```python
from build123d import *

# Parameters (mm, degrees)
SKETCH_1_R          = 30
EXTRUDE_1_DEPTH     = 10
CUT_EXTRUDE_1_REACH = 45.589
SKETCH_2_R          = 1.8
SKETCH_3_R          = 3.25
CUT_EXTRUDE_2_DEPTH = 5
CUT_EXTRUDE_3_REACH = 45.589
SKETCH_4_R          = 1.8
SKETCH_5_R          = 3.15
CUT_EXTRUDE_4_DEPTH = 3
CUT_EXTRUDE_5_REACH = 45.589
SKETCH_6_R          = 11
CUT_EXTRUDE_START   = -5
CUT_EXTRUDE_6_DEPTH = 5


# Read off the part's stored shape, not the designer's step: 切除-拉伸6
with BuildPart() as part:
    # 草图1 → 凸台-拉伸1 (new body)
    with BuildSketch(Plane.XY):
        Circle(SKETCH_1_R)
    extrude(amount=EXTRUDE_1_DEPTH)

    # 草图2 → 切除-拉伸1 (cut, up to next)
    with BuildSketch(Plane.XY.offset(10), mode=Mode.PRIVATE) as cut_extrude_1_sk1:
        with Locations((0, 14)):
            Circle(SKETCH_2_R)
    cut_extrude_1_tool1 = extrude(cut_extrude_1_sk1.sketch, amount=-CUT_EXTRUDE_1_REACH, mode=Mode.PRIVATE) & part.part
    # 草图2 → 切除-拉伸1 (cut, up to next)
    with BuildSketch(Plane.XY.offset(10), mode=Mode.PRIVATE) as cut_extrude_1_sk2:
        with Locations((12.124355653, -7)):
            Circle(SKETCH_2_R)
    cut_extrude_1_tool2 = extrude(cut_extrude_1_sk2.sketch, amount=-CUT_EXTRUDE_1_REACH, mode=Mode.PRIVATE) & part.part
    # 草图2 → 切除-拉伸1 (cut, up to next)
    with BuildSketch(Plane.XY.offset(10), mode=Mode.PRIVATE) as cut_extrude_1_sk3:
        with Locations((-12.124355653, -7)):
            Circle(SKETCH_2_R)
    cut_extrude_1_tool3 = extrude(cut_extrude_1_sk3.sketch, amount=-CUT_EXTRUDE_1_REACH, mode=Mode.PRIVATE) & part.part
    add(cut_extrude_1_tool1.solids().sort_by_distance((0, 14, 10))[0], mode=Mode.SUBTRACT)
    add(cut_extrude_1_tool2.solids().sort_by_distance((12.124356, -7, 10))[0], mode=Mode.SUBTRACT)
    add(cut_extrude_1_tool3.solids().sort_by_distance((-12.124356, -7, 10))[0], mode=Mode.SUBTRACT)

    # 草图3 → 切除-拉伸2 (cut)
    with BuildSketch(Plane(origin=(0, 0, 0), x_dir=(-1, 0, 0), z_dir=(0, 0, -1))):
        with Locations((0, 14)):
            Circle(SKETCH_3_R)
        with Locations((12.125855653, -6.999133975)):
            Circle(SKETCH_3_R)
        with Locations((-12.122855653, -7.000866025)):
            Circle(SKETCH_3_R)
    extrude(amount=-CUT_EXTRUDE_2_DEPTH, mode=Mode.SUBTRACT)

    # 草图4 → 切除-拉伸3 (cut, up to next)
    with BuildSketch(Plane.XY.offset(10), mode=Mode.PRIVATE) as cut_extrude_3_sk1:
        with Locations((-15, -20)):
            Circle(SKETCH_4_R)
    cut_extrude_3_tool1 = extrude(cut_extrude_3_sk1.sketch, amount=-CUT_EXTRUDE_3_REACH, mode=Mode.PRIVATE) & part.part
    # 草图4 → 切除-拉伸3 (cut, up to next)
    with BuildSketch(Plane.XY.offset(10), mode=Mode.PRIVATE) as cut_extrude_3_sk2:
        with Locations((15, -20)):
            Circle(SKETCH_4_R)
    cut_extrude_3_tool2 = extrude(cut_extrude_3_sk2.sketch, amount=-CUT_EXTRUDE_3_REACH, mode=Mode.PRIVATE) & part.part
    # 草图4 → 切除-拉伸3 (cut, up to next)
    with BuildSketch(Plane.XY.offset(10), mode=Mode.PRIVATE) as cut_extrude_3_sk3:
        with Locations((15, 20)):
            Circle(SKETCH_4_R)
    cut_extrude_3_tool3 = extrude(cut_extrude_3_sk3.sketch, amount=-CUT_EXTRUDE_3_REACH, mode=Mode.PRIVATE) & part.part
    # 草图4 → 切除-拉伸3 (cut, up to next)
    with BuildSketch(Plane.XY.offset(10), mode=Mode.PRIVATE) as cut_extrude_3_sk4:
        with Locations((-15, 20)):
            Circle(SKETCH_4_R)
    cut_extrude_3_tool4 = extrude(cut_extrude_3_sk4.sketch, amount=-CUT_EXTRUDE_3_REACH, mode=Mode.PRIVATE) & part.part
    add(cut_extrude_3_tool1.solids().sort_by_distance((-15, -20, 10))[0], mode=Mode.SUBTRACT)
    add(cut_extrude_3_tool2.solids().sort_by_distance((15, -20, 10))[0], mode=Mode.SUBTRACT)
    add(cut_extrude_3_tool3.solids().sort_by_distance((15, 20, 10))[0], mode=Mode.SUBTRACT)
    add(cut_extrude_3_tool4.solids().sort_by_distance((-15, 20, 10))[0], mode=Mode.SUBTRACT)

    # 草图5 → 切除-拉伸4 (cut)
    with BuildSketch(Plane.XY.offset(10)):
        with Locations((-15, 20)):
            Circle(SKETCH_5_R)
        with Locations((15, 20)):
            Circle(SKETCH_5_R)
        with Locations((15, -20)):
            Circle(SKETCH_5_R)
        with Locations((-15, -20)):
            Circle(SKETCH_5_R)
    extrude(amount=-CUT_EXTRUDE_4_DEPTH, mode=Mode.SUBTRACT)

    # 草图6 → 切除-拉伸5 (cut, up to next)
    with BuildSketch(Plane.XY.offset(10), mode=Mode.PRIVATE) as cut_extrude_5_sk1:
        Circle(SKETCH_6_R)
    cut_extrude_5_tool1 = extrude(cut_extrude_5_sk1.sketch, amount=-CUT_EXTRUDE_5_REACH, mode=Mode.PRIVATE) & part.part
    add(cut_extrude_5_tool1.solids().sort_by_distance((0, 0, 10))[0], mode=Mode.SUBTRACT)

    # 切除-拉伸6 outline → 切除-拉伸6 (cut)
    with BuildSketch(Plane(origin=(0, 0, 0), x_dir=(-1, 0, 0), z_dir=(0, 0, -1)).offset(CUT_EXTRUDE_START)):
        with BuildLine():
            Line((-10.725995825, -2.439879827), (-13.749355653, -4.185417438))
            ThreePointArc((-13.749355653, -4.185417438), (-15.374355624, -7.000433013), (-13.748605595, -9.815015475))
            ThreePointArc((-13.748605595, -9.815015475), (-14.784005692, -5.135181039), (-10.031538938, -4.513117164))
            ThreePointArc((-10.031538938, -4.513117164), (-10.430407021, -3.493795841), (-10.725995825, -2.439879827))
        make_face()
        with BuildLine():
            Line((-3.25, 14), (-3.25, 10.508924778))
            ThreePointArc((-3.25, 10.508924778), (-2.189145313, 10.779964879), (-1.10660044, 10.944196429))
            ThreePointArc((-1.10660044, 10.944196429), (-2.660728418, 12.133713772), (-3.25, 14))
        make_face()
        with BuildLine():
            ThreePointArc((-8.92286522, -6.432921286), (-9.15608578, -8.327808571), (-10.413102364, -9.764784202))
            Line((-10.413102364, -9.764784202), (-7.475995825, -8.069044952))
            ThreePointArc((-7.475995825, -8.069044952), (-8.240138715, -7.2869825), (-8.92286522, -6.432921286))
        make_face()
        with BuildLine():
            Line((3.25, 10.508924778), (3.25, 14))
            ThreePointArc((3.25, 14), (2.660728418, 12.133713772), (1.10660044, 10.944196429))
            ThreePointArc((1.10660044, 10.944196429), (2.189145313, 10.779964879), (3.25, 10.508924778))
        make_face()
        with BuildLine():
            ThreePointArc((8.926440063, -6.427959847), (8.242163905, -7.284691768), (7.475995825, -8.069044952))
            Line((7.475995825, -8.069044952), (10.499355653, -9.814582562))
            ThreePointArc((10.499355653, -9.814582562), (12.124788665, -10.249999971), (13.750105595, -9.81414945))
            ThreePointArc((13.750105595, -9.81414945), (10.258542955, -9.659142113), (8.926440063, -6.427959847))
        make_face()
        with BuildLine():
            ThreePointArc((10.725995825, -2.439879827), (10.430184526, -3.49446001), (10.030964095, -4.514394681))
            ThreePointArc((10.030964095, -4.514394681), (11.789659007, -3.766569697), (13.664602363, -4.136485104))
            Line((13.664602363, -4.136485104), (10.725995825, -2.439879827))
        make_face()
    extrude(amount=CUT_EXTRUDE_6_DEPTH, mode=Mode.SUBTRACT)


solid = part.part
```
Source: CAD feature listing. Evaluate the final solid. Frame: model axes, mm. A direction names the side the tool comes from. Give positions to 0.01 mm unless a question says otherwise; leave off trailing zeros. Write each loop counter-clockwise with the first axis right and the second up, starting at its lowest first coordinate (ties: lowest second). Pieces come first, ordered by that corner, then holes. Notation, with made-up numbers: (12, 82.25) - (61, 82.25) arc R34 cw to (61, 113.25) - close; hole circle Ø9 at (9.5, -17). An arc over 180 degrees is marked (long way). One line per item, written item: value. Start each with the question number.
Q1. Section query C-C, the plane y = 20. Return the cut outline in (x, z), then the cut area to 3 significant figures.
Q2. Section query B-B, the plane y = 0. Return the cut outline in (x, z), then the cut area to 3 significant figures.
Q3. Section query D-D, the plane x = -22. Return the cut outline in (y, z).
Q4. Section query A-A, the plane z = 6. Count the separate pieces of the cut face and the enclosed holes in it, then the cut area to 3 significant figures.
Q5. Set-up query: faces 1 (the face through (-1, 12, 5)), 2 (the face through (-18.147, 20.138, 8.521)), 3 (the face through (13, 0, 10)). Return all of +Z, -Z, +X, -X, +Y, -Y with unobstructed straight access to the full face (end or side cutting, diameter ignored); none if empty.
Q6. Material intervals for probe 1 along Y at (x, z) = (0, 6.9); probe 2 along Y at (x, z) = (0, 3.5); probe 3 along Y at (x, z) = (-15, 5.75), sorted ascending. Write a range as from..to.
Q7. First-contact query: pin 1 Ø1 at (x, y) = (-16, -5.5) entering from -Z; pin 2 Ø2 at (x, z) = (0, 7) entering from +Y; pin 3 Ø4 at (y, z) = (11.5, 3.5) entering from -X; pin 4 Ø4 at (y, z) = (23, 6.5) entering from +X. Flat tips, straight axial feed; report the tip coordinate or a pass-through.
Q8. Draft query along X for faces 4 (the face through (-18.147, -19.862, 8.521)), 5 (the face through (13, 0, 0)), 6 (the face through (-29.97, 1.32, 4.93)). Return one class per face: +X half, -X half, draft (parallel to the pull), parting line (faces both ways), or undercut.
Answer:
1. outline: (-22.36, 0) - (-16.8, 0) - (-16.8, 7) - (-18.15, 7) - (-18.15, 10) - (-22.36, 10) - close; (-13.2, 0) - (13.2, 0) - (13.2, 7) - (11.85, 7) - (11.85, 10) - (-11.85, 10) - (-11.85, 7) - (-13.2, 7) - close; (16.8, 0) - (22.36, 0) - (22.36, 10) - (18.15, 10) - (18.15, 7) - (16.8, 7) - close
1. area: 359 mm2
2. outline: (-30, 0) - (-11, 0) - (-11, 10) - (-30, 10) - close; (11, 0) - (30, 0) - (30, 10) - (11, 10) - close
2. area: 380 mm2
3. outline: (-20.4, 0) - (20.4, 0) - (20.4, 10) - (-20.4, 10) - close
4. separate pieces: 1
4. enclosed holes: 8
4. area: 2,380 mm2
5. face 1: -Z
5. face 2: +Z
5. face 3: +Z, +X, -X, +Y, -Y
6. probe 1: y = -30..-11, 11..12.2, 15.8..30
6. probe 2: y = -30..-11, 17.25..30
6. probe 3: y = -25.98..-21.8, -18.2..18.2, 21.8..25.98
7. pin 1: stops at z = 0
7. pin 2: stops at y = 30
7. pin 3: stops at x = -28.46
7. pin 4: stops at x = 21.42
8. face 4: undercut
8. face 5: draft
8. face 6: parting line
